Model file for the job. Use its own axes, mm. Face numbers are marked on the shaded views. A direction names the side the tool comes from. Give positions to 0.01 mm unless a question says otherwise; leave off trailing zeros. Write each loop counter-clockwise with the first axis right and the second up, starting at its lowest first coordinate (ties: lowest second). Pieces come first, ordered by that corner, then holes. Notation, with made-up numbers: M -13.5,-22.5 L -5.5,-22.5 A26 cw -5.5,8.5 Z; hole C 23,-5 d4. An arc over 180 degrees is marked long. Answer as a JSON object with one key per item and string values. Group by question number.
```python
from build123d import *

# Parameters (mm, degrees)
SKETCH1_W           = 50.8
SKETCH1_H           = 25.4
BOSS_EXTRUDE1_DEPTH = 6.35
BOSS_EXTRUDE2_DEPTH = 3.175
SKETCH3_R           = 2.2225
BOSS_EXTRUDE3_DEPTH = 6.35


with BuildPart() as part:
    # Sketch1 → Boss-Extrude1 (new, symmetric)
    with BuildSketch(Plane(origin=(0, 0, 0), x_dir=(1, 0, 0), z_dir=(0, 1, 0))):
        Rectangle(SKETCH1_W, SKETCH1_H)
    extrude(amount=BOSS_EXTRUDE1_DEPTH, both=True)

    # Sketch2 → Boss-Extrude2 (add, symmetric)
    with BuildSketch(Plane(origin=(0, 0, 0), x_dir=(1, 0, 0), z_dir=(0, 1, 0))):
        with BuildLine():
            Line((-25.4, 3.175), (-27.051, 3.175))
            Line((-27.051, 3.175), (-33.655, 0.635))
            Line((-33.655, 0.635), (-33.655, -1.04))
            Line((-33.655, -1.04), (-27.94, -1.04))
            ThreePointArc((-27.94, -1.04), (-26.44, -2.54), (-27.94, -4.04))
            Line((-27.94, -4.04), (-33.655, -4.04))
            Line((-33.655, -4.04), (-33.655, -5.715))
            Line((-33.655, -5.715), (-27.051, -8.255))
            Line((-27.051, -8.255), (-25.4, -8.255))
            Line((-25.4, -8.255), (-25.4, 3.175))
        make_face()
        with BuildLine():
            Line((25.4, 3.175), (25.4, -8.255))
            Line((25.4, -8.255), (27.051, -8.255))
            Line((27.051, -8.255), (33.655, -5.715))
            Line((33.655, -5.715), (33.655, -4.04))
            Line((33.655, -4.04), (27.94, -4.04))
            ThreePointArc((27.94, -4.04), (26.44, -2.54), (27.94, -1.04))
            Line((27.94, -1.04), (33.655, -1.04))
            Line((33.655, -1.04), (33.655, 0.635))
            Line((33.655, 0.635), (27.051, 3.175))
            Line((27.051, 3.175), (25.4, 3.175))
        make_face()
    extrude(amount=BOSS_EXTRUDE2_DEPTH, both=True)

    # Sketch3 → Boss-Extrude3 (add, symmetric)
    with BuildSketch(Plane.XY.offset(12.7)):
        with Locations(Location((-3.81, 0, 0), (0, 0, 180))):
            Circle(SKETCH3_R)
        with Locations(Location((-11.43, 0, 0), (0, 0, 180))):
            Circle(SKETCH3_R)
        with Locations(Location((11.43, 0, 0), (0, 0, 180))):
            Circle(SKETCH3_R)
        with Locations(Location((3.81, 0, 0), (0, 0, 180))):
            Circle(SKETCH3_R)
    extrude(amount=BOSS_EXTRUDE3_DEPTH, both=True)


solid = part.part
```
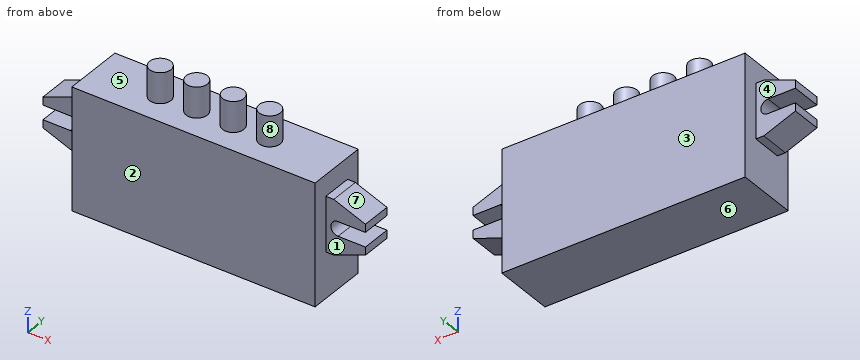
Q1. 3-axis set-ups, long thin cutter, end or side, ignore diameter. For the marked faces 1, 2, 3, 4 and 5: which of +Z, -Z, +X, -X, +Y, -Y reach the whole face in a straight line?
Q2. Wall check: L1, parallel to X at y = 1.25, z = 17.5; L2, parallel to Z at x = -18.5, y = -2.75; L3, parallel to X at y = 5.25, z = 10.5. Give the ranges that are in metal, low to high.
Q3. Drop flat-ended pins along their axis: P1, Ø0.5, axis at x = -26.5, y = 1, coming from the -Z side (3 decimals); P2, Ø0.5, axis at x = 26.5, y = 1.5, coming from the +Z side (3 decimals); P3, Ø3, axis at x = -31, y = -0.5, coming from the +Z side. Give the stop position or say it passes through.
Q4. Slice it at D-D, the plane z = 14.5. Write the cut outline in (x, y) (1 decimal).
Q5. Two-plate mould, pull along X, no slides. Class the marked faces 6, 7 and 8: +X half, -X half, draft (parallel to the pull), parting line (faces both ways), or undercut.
Q6. Slice it at C-C, the plane y = 4.5. Write the cut outline in (x, z), then the cut area to 3 significant figures.
Q7. Slice it at B-B, the plane z = -2.5. Write the cut outline in (x, y) (3 decimals), then the cut area to 3 significant figures.
Q8. Slice it at A-A, the plane x = -3.81. Write the cut outline in (y, z).
Solved:
{
 "1": {"face 1": "+Z, -Z, +X, -Y", "face 2": "+Z, -Z, +X, -X, -Y", "face 3": "+Z, -Z, +X, -X, +Y", "face 4": "+Z, -Z, -X, +Y", "face 5": "+Z"},
 "2": {"L1": "x = -13.27 to -9.59, -5.65 to -1.97, 1.97 to 5.65, 9.59 to 13.27", "L2": "z = -12.7 to 12.7", "L3": "x = -25.4 to 25.4"},
 "3": {"P1": "stops at z = -3.175", "P2": "stops at z = 8.255", "P3": "stops at z = 7.31"},
 "4": {"outline": "C -11.4,0 d4.4; C -3.8,0 d4.4; C 3.8,0 d4.4; C 11.4,0 d4.4"},
 "5": {"face 6": "draft", "face 7": "+X half", "face 8": "undercut"},
 "6": {"outline": "M -25.4,-12.7 L 25.4,-12.7 L 25.4,12.7 L -25.4,12.7 Z", "area": "1,290 mm²"},
 "7": {"outline": "M -28.806,-3.175 L -25.4,-3.175 L -25.4,-6.35 L 25.4,-6.35 L 25.4,-3.175 L 28.806,-3.175 L 28.806,3.175 L 25.4,3.175 L 25.4,6.35 L -25.4,6.35 L -25.4,3.175 L -28.806,3.175 Z", "area": "688 mm²"},
 "8": {"outline": "M -6.35,-12.7 L 6.35,-12.7 L 6.35,12.7 L 2.22,12.7 L 2.22,19.05 L -2.22,19.05 L -2.22,12.7 L -6.35,12.7 Z"}
}
